Check sheet for the drawn part. Datum: minimum x, y, z corner. Units: mm. A direction names the side the tool comes from. Coordinates: 2 decimals unless noted, no trailing zeros. Write each loop counter-clockwise with the first axis right and the second up, starting at its lowest first coordinate (ties: lowest second). Pieces come first, ordered by that corner, then holes. Notation, with made-up numbers: (45, 43) -> (96, 43) arc R14 cw to (96, 67) -> close; hole circle Ø1 at (80, 55). An arc over 180 degrees is marked (long way). Write item = value, one per line. Start each with the question number.
(1) Material ranges on probe 1 along Y at (x, z) = (25, 10.5); probe 2 along Z at (x, y) = (19, 23.5), recorded low to high. Write a range as [from, to].
(2) Section check A-A (z = 10.75). Record the cut outline in (x, y).
(3) Mould release check, pull along X, two halves, no side actions. Record for the marked faces 5, 6 and 7: released by +X, released by -X, zero draft, split by the parting line, or undercut.
(4) Section check B-B (y = 15). Record the cut outline in (x, z), plus the area to 4 significant figures.
(5) Set-up check for the marked faces 1, 2, 3 and 4: record each of +Z, -Z, +X, -X, +Y, -Y from which the full face is reachable in a straight line by a thin tool's end or side.
(6) Gauge pin test, flat ends, axial feed: pin 1 Ø2 at (x, y) = (10, 19) entering from +Z; pin 2 Ø3 at (x, z) = (27.5, 9) entering from -Y; pin 3 Ø2 at (y, z) = (35, 5.5) entering from -X. Record the tip position at first contact, or that the pin passes through.
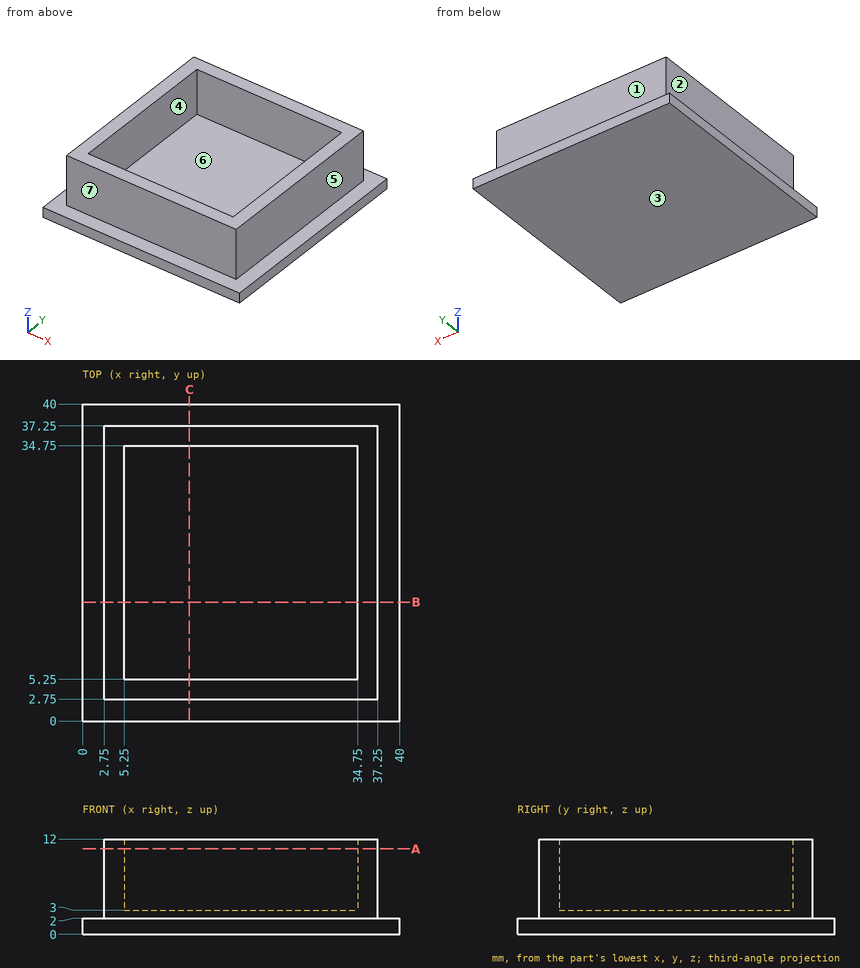
Response:
q1.probe_1 = [2.75, 5.25], [34.75, 37.25]
q1.probe_2 = [0, 3]
q2.outline = (2.75, 2.75) -> (37.25, 2.75) -> (37.25, 37.25) -> (2.75, 37.25) -> close; hole (5.25, 5.25) -> (34.75, 5.25) -> (34.75, 34.75) -> (5.25, 34.75) -> close
q3.face_5 = released by +X
q3.face_6 = undercut
q3.face_7 = zero draft
q4.outline = (0, 0) -> (40, 0) -> (40, 2) -> (37.25, 2) -> (37.25, 12) -> (34.75, 12) -> (34.75, 3) -> (5.25, 3) -> (5.25, 12) -> (2.75, 12) -> (2.75, 2) -> (0, 2) -> close
q4.area = 159.5 mm2
q5.face_1 = +Z, +X, -X, +Y
q5.face_2 = +Z, -X, +Y, -Y
q5.face_3 = -Z, +X, -X, +Y, -Y
q5.face_4 = +Z
q6.pin_1 = 3
q6.pin_2 = 2.75
q6.pin_3 = 2.75
